Geometry: see drawing. Coordinates: mm, zero at the bounding-box minimum. Coordinates: 2 decimals unless noted, no trailing zeros. Write each loop counter-clockwise with the first axis right and the second up, starting at its lowest first coordinate (ties: lowest second). Pieces come first, ordered by that corner, then holes. Notation, with made-up numbers: (33, -35.75) - (42, -35.75) arc R15 ccw to (42, -13.75) - close; hole circle Ø1 at (11, 82.25). An arc over 180 degrees is marked (long way). One line per question, with ' | ' between items. Start each with the question number.
Q1. Cut plane A-A, the plane z = 74. Return loops of the section in (x, y) (1 decimal).
Q2. Line query: line 1 (X direction, y = 3, z = 72.5); line 2 (X direction, y = 2, z = 25); line 3 (X direction, y = 7, z = 74.5). Output: solid intervals per line, ascending.
Q3. Contact query for flat-ended pins moving along their axis: P1, Ø6, axis at x = 114.3, z = 72.91, coming from the +Y side; P2, Ø7.5, axis at x = 114.3, z = 22.44, coming from the -Y side. Output: stop coordinate, or through.
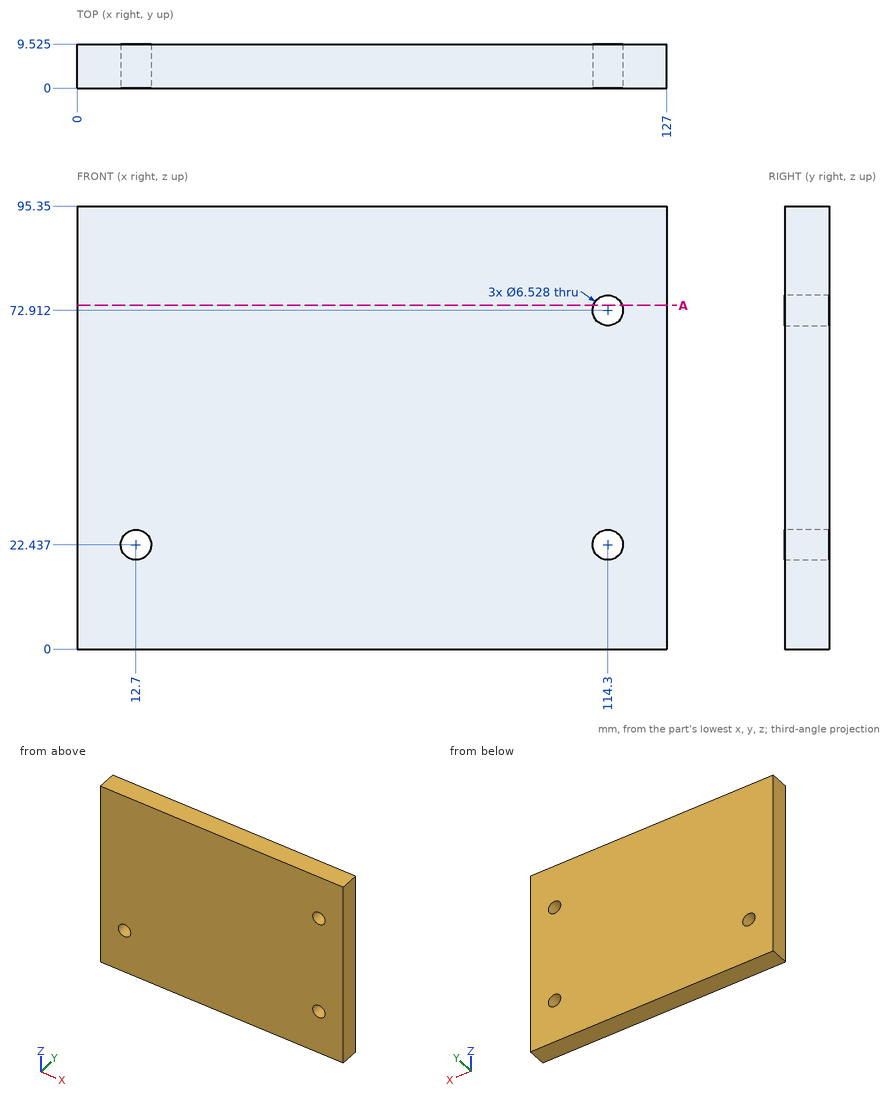
Reply:
1) outline: (0, 0) - (111.2, 0) - (111.2, 9.5) - (0, 9.5) - close; (117.4, 0) - (127, 0) - (127, 9.5) - (117.4, 9.5) - close
2) line 1: x = 0 to 111.06, 117.54 to 127 | line 2: x = 0 to 10.68, 14.72 to 112.28, 116.32 to 127 | line 3: x = 0 to 111.45, 117.15 to 127
3) P1: passes through | P2: stops at y = 0
